Source: CAD feature listing. Evaluate the final solid. Frame: model axes, mm. A direction names the side the tool comes from. Round coordinates to 2 decimals unless told otherwise and drop trailing zeros. Order: outer loops, then holes, each group sorted by start corner. A loop starts at its lowest first (then second) coordinate and runs counter-clockwise, first axis right, second up. Notation, with made-up numbers: M 76.25,5.25 L 104.25,5.25 A14 cw 104.25,12.25 Z; hole C 85.5,74 d9. An arc over 180 degrees is marked long. Answer in a Markdown table with one row per item. Add a question column.
```python
from build123d import *

# Parameters (mm, degrees)
SKETCH2_W               = 41.746000074
SKETCH2_H               = 9.873000066
BOSS_EXTRUDE1_DEPTH     = 3.746000128
SKETCH3_W               = 23.746000006
SKETCH3_H               = 9.873000066
BOSS_EXTRUDE2_DEPTH     = 6.548499984
FILLET1_R               = 5.0165
SKETCH4_R               = 2.99974
CUT_EXTRUDE1_DEPTH      = 26.281119307
CUT_EXTRUDE2_DEPTH      = 23.426190384
CUT_EXTRUDE2_DEPTH_BACK = 2.54
SKETCH6_R               = 0.508
SKETCH7_R               = 0.508
CUT_EXTRUDE3_DEPTH      = 2.54


with BuildPart() as part:
    # Sketch2 → Boss-Extrude1 (new body)
    with BuildSketch(Plane(origin=(0, 0, 0), x_dir=(1, 0, 0), z_dir=(0, 1, 0))):
        Rectangle(SKETCH2_W, SKETCH2_H)
    extrude(amount=BOSS_EXTRUDE1_DEPTH)

    # Sketch3 → Boss-Extrude2 (add)
    with BuildSketch(Plane(origin=(0, 3.746000128, 0), x_dir=(1, 0, 0), z_dir=(0, 1, 0))):
        with Locations((-0.00733485, 0)):
            Rectangle(SKETCH3_W, SKETCH3_H)
    extrude(amount=BOSS_EXTRUDE2_DEPTH)

    # Fillet1
    fillet1_edges = [part.edges().sort_by_distance(p)[0] for p in [
        (-11.880334853, 3.746000128, 0),
        (11.865665153, 3.746000128, 0),
    ]]
    fillet(fillet1_edges, radius=FILLET1_R)

    # Sketch4 → Cut-Extrude1 (cut, through all)
    with BuildSketch(Plane.XY.offset(4.936500033)):
        with Locations((-0.00733485, 10.294500112)):
            Circle(SKETCH4_R)
    extrude(amount=-CUT_EXTRUDE1_DEPTH, mode=Mode.SUBTRACT)

    # Sketch6 → Cut-Extrude2 (cut, two sides: drawn at the far end of the back side and taken through both)
    with BuildSketch(Plane(origin=(0, 3.746000128, 0), x_dir=(1, 0, 0), z_dir=(0, 1, 0)).offset(-CUT_EXTRUDE2_DEPTH_BACK)):
        with Locations(Location((-16.896834853, 0, 0), (0, 0, 270))):
            Circle(SKETCH6_R)
        with Locations(Location((16.896834853, 0, 0), (0, 0, 90))):
            Circle(SKETCH6_R)
    extrude(amount=CUT_EXTRUDE2_DEPTH + CUT_EXTRUDE2_DEPTH_BACK, mode=Mode.SUBTRACT)

    # Sketch7 → Cut-Extrude3 (cut)
    with BuildSketch(Plane(origin=(0, 10.294500112, 0), x_dir=(1, 0, 0), z_dir=(0, 1, 0))):
        with Locations(Location((-6.99999997, 0, 0), (0, 0, 270))):
            Circle(SKETCH7_R)
        with Locations(Location((6.99999997, 0, 0), (0, 0, 90))):
            Circle(SKETCH7_R)
    extrude(amount=-CUT_EXTRUDE3_DEPTH, mode=Mode.SUBTRACT)


solid = part.part
```
(1) Pin query (flat end, axial travel): pin 1 (1.7 mm diameter, centred on y = 9.5, z = -1.5, fed in from -X); pin 2 (0.8 mm diameter, centred on x = 7, z = 0, fed in from +Y); pin 3 (1.2 mm diameter, centred on x = -18, z = 2, fed in from +Y). Return the tip coordinate at first contact, or that it passes through.
(2) Line query: line 1 (X direction, y = 2.5, z = 0); line 2 (X direction, y = 8.5, z = 0.25); line 3 (Z direction, x = 7, y = 9.25). Output: solid intervals per line, ascending. Write a range as from..to.
(3) Cut plane D-D (y = 6.5). Return loops of the section in (x, z), and give its area (3 significant figures).
(4) Cut plane B-B (x = -7). Return loops of the section in (y, z), and give its area (3 significant figures).
(5) Cut plane A-A (z = 0). Return loops of the section in (x, y).
(6) Draft query along Z for faces 1 (the face through (-16.4, 2.5, -0.1)), 2 (the face through (16.4, 2.5, 0.1)), 3 (the face through (0, 4, 4.937)), 4 (the face through (-8, 10.295, 0)). Return one class per face: +Z half, -Z half, draft (parallel to the pull), parting line (faces both ways), or undercut.
(7) Cut plane C-C (z = 3.5). Return loops of the section in (x, y).
(8) Access query for faces 5 (the face through (0, 0, 0)), 6 (the face through (-19, 3.746, 0)), 7 (the face through (0, 4, -4.937)), 8 (the face through (11.866, 10, 0)), 9 (the face through (7, 7.755, 0)). Directions: +Z, -Z, +X, -X, +Y, -Y. A direction counts if a zero-diameter tool reaches every point of the face in a straight line with its end or side. Return the directions, or none.
Answer list:
| question | item | result |
|---|---|---|
| 1 | pin 1 | x = -11.88 |
| 1 | pin 2 | y = 7.75 |
| 1 | pin 3 | y = 3.75 |
| 2 | line 1 | -20.87..-17.4, -16.39..16.39, 17.4..20.87 |
| 2 | line 2 | -11.89..-7.44, -6.56..-2.41, 2.4..6.56, 7.44..11.87 |
| 2 | line 3 | -4.94..-0.51, 0.51..4.94 |
| 3 | outline | M -12.42,-4.94 L 12.4,-4.94 L 12.4,4.94 L -12.42,4.94 Z |
| 3 | area | 245 mm² |
| 4 | outline | M 0,-4.94 L 10.29,-4.94 L 10.29,-0.51 L 7.75,-0.51 L 7.75,0.51 L 10.29,0.51 L 10.29,4.94 L 0,4.94 Z |
| 4 | area | 99.1 mm² |
| 5 | outline | M -20.87,0 L 20.87,0 L 20.87,3.75 L 17.4,3.75 L 17.4,1.21 L 16.39,1.21 L 16.39,3.77 A5.02 cw 11.87,8.76 L 11.87,10.29 L 7.51,10.29 L 7.51,7.75 L 6.49,7.75 L 6.49,10.29 L 2.99,10.29 A3 cw -3.01,10.29 L -6.49,10.29 L -6.49,7.75 L -7.51,7.75 L -7.51,10.29 L -11.88,10.29 L -11.88,8.76 A5.02 cw -16.39,3.77 L -16.39,1.21 L -17.4,1.21 L -17.4,3.75 L -20.87,3.75 Z |
| 6 | face 1 | undercut |
| 6 | face 2 | undercut |
| 6 | face 3 | +Z half |
| 6 | face 4 | draft |
| 7 | outline | M -20.87,0 L 20.87,0 L 20.87,3.75 L 16.88,3.75 A5.02 cw 11.87,8.76 L 11.87,10.29 L 2.99,10.29 A3 cw -3.01,10.29 L -11.88,10.29 L -11.88,8.76 A5.02 cw -16.9,3.75 L -20.87,3.75 Z |
| 8 | face 5 | +Z, -Z, +X, -X, -Y |
| 8 | face 6 | +Z, -Z, -X, +Y |
| 8 | face 7 | -Z, +X, -X, +Y, -Y |
| 8 | face 8 | +Z, -Z, +X, +Y |
| 8 | face 9 | +Y |
